Build history of the part. All positions in model axes, mm. A direction names the side the tool comes from. Coordinates: 2 decimals unless noted, no trailing zeros. Write each loop counter-clockwise with the first axis right and the second up, starting at its lowest first coordinate (ties: lowest second). Pieces come first, ordered by that corner, then holes. Notation, with made-up numbers: (16, 25) -> (57, 25) arc R25 cw to (57, 48) -> close; hole circle Ø1 at (73, 50.25). An arc over 180 degrees is marked (long way). Write each question's results on one line, items separated by ' | '. Start each with the question number.
Q1. Drop flat-ended pins along their axis: pin 1 Ø1.2 at (x, z) = (-10, 4) entering from -Y; pin 2 Ø4.5 at (x, y) = (-10.5, 7) entering from +Z; pin 3 Ø2 at (x, z) = (-3.5, 0.5) entering from +Y. Give the stop position or say it passes through.
Q2. Saw through at C-C on y = 1.5. Give the cut face in (x, z), and give its area (3 significant figures).
Q3. Drill centre lines: line 1 (Z direction, x = -1.25, y = 3.5); line 2 (Z direction, x = -14, y = 35); line 3 (Y direction, x = -9, z = -4). Where is each one in solid material? Low to high.
Q4. Tool access for faces 4 (the face through (-7.395, -9.491, 2.915)), 5 (the face through (-7, 4, 4.906)), 6 (the face through (0, -16, -3.3)): list every direction of +Z, -Z, +X, -X, +Y, -Y with a clear straight run to the whole face (end or side of a thin tool).
Q5. Two-plate mould, pull along Y, no slides. Class faces 1 (the face through (-7, 4, 3.406)), 2 (the face through (-7, 28, 2.406)), 3 (the face through (-7, -56.781, -5)): released by +Y, released by -Y, zero draft, split by the parting line, or undercut.
Q6. Saw through at D-D on z = -0.75. Give the cut face in (x, y).
Q7. Saw through at B-B on y = 20. Give the cut face in (x, z), and give its area (3 significant figures).
from build123d import *

# Parameters (mm, degrees)
F1_DEPTH = 15
F2_R     = 5
F3_W     = 19
F3_H     = 3.5
F4_DEPTH = 25
F5_R     = 5
F6_R     = 0.99999


# Not quite as in the source:
# - a fillet or chamfer is up to 0.001 mm smaller than in the source, because OpenCascade refuses the exact size


with BuildPart() as f1:
    # F0 (on Right) → F1 (new body)
    with BuildSketch(Plane.YZ):
        with BuildLine():
            Line((15.2185663986, 4.9061592609), (-8.3786299068, 4.9061592609))
            ThreePointArc((-8.3786299068, 4.9061592609), (-10.2743175345, 4.4284267718), (-11.7171893777, 3.10934347))
            Line((-11.7171893777, 3.10934347), (-15.1529792105, -2.0970249483))
            ThreePointArc((-15.1529792105, -2.0970249483), (-16.5958510537, -3.41610825), (-18.4915386814, -3.8938407391))
            Line((-18.4915386814, -3.8938407391), (-56.7814336014, -3.8938407391))
            Line((-56.7814336014, -3.8938407391), (-56.7814336014, -5.3938407391))
            Line((-56.7814336014, -5.3938407391), (-17.6842372959, -5.3938407391))
            ThreePointArc((-17.6842372959, -5.3938407391), (-15.7885496683, -4.91610825), (-14.3456778251, -3.5970249483))
            Line((-14.3456778251, -3.5970249483), (-10.9098879922, 1.60934347))
            ThreePointArc((-10.9098879922, 1.60934347), (-9.467016149, 2.9284267718), (-7.5713285214, 3.4061592609))
            Line((-7.5713285214, 3.4061592609), (15.2185663986, 3.4061592609))
            Line((15.2185663986, 3.4061592609), (15.2185663986, 4.9061592609))
        make_face()
    extrude(amount=-F1_DEPTH)

    # F2
    f2_edges = [f1.edges().sort_by_distance(p)[0] for p in [
        (-15, -56.781434, -4.643841),
        (0, -56.781434, -4.643841),
    ]]
    fillet(f2_edges, radius=F2_R)

    # F3 (on face) → F4 (join)
    with BuildSketch(Plane(origin=(0, 15.2185663986, 0), x_dir=(-1, 0, 0), z_dir=(0, 1, 0))):
        with Locations((7.5, 4.1561592609)):
            Rectangle(F3_W, F3_H)
    extrude(amount=F4_DEPTH)

    # F5
    f5_edges = [f1.edges().sort_by_distance(p)[0] for p in [
        (2, 40.218566, 4.156159),
        (-17, 40.218566, 4.156159),
    ]]
    fillet(f5_edges, radius=F5_R)

    # F6 (radius 1 in the source; OpenCascade refuses exactly that, so slightly less here)
    f6_edges = [f1.edges().sort_by_distance(p)[0] for p in [
        (-17, 25.218566, 5.906159),
        (-15.535534, 38.7541, 5.906159),
        (-7.5, 15.218566, 5.906159),
        (-7.5, 40.218566, 5.906159),
        (2, 25.218566, 5.906159),
        (0.535534, 38.7541, 5.906159),
        (2, 25.218566, 2.406159),
        (0.535534, 38.7541, 2.406159),
        (-7.5, 15.218566, 2.406159),
        (-7.5, 40.218566, 2.406159),
        (-17, 25.218566, 2.406159),
        (-15.535534, 38.7541, 2.406159),
        (2, 15.218566, 4.156159),
        (-17, 15.218566, 4.156159),
    ]]
    fillet(f6_edges, radius=F6_R)


solid = f1.part
Returned:
1) pin 1: stops at y = -11.51 | pin 2: stops at z = 4.91 | pin 3: stops at y = -10.98
2) outline: (-15, 3.41) -> (0, 3.41) -> (0, 4.91) -> (-15, 4.91) -> close | area: 22.5 mm2
3) line 1: z = 3.41 to 4.91 | line 2: z = 2.41 to 5.91 | line 3: y = -56.78 to -14.65
4) face 4: -Z, +X, -X | face 5: +Z, +X, -X, -Y | face 6: +Z, -Z, +X, -Y
5) face 1: undercut | face 2: zero draft | face 3: released by -Y
6) outline: (-15, -14.26) -> (0, -14.26) -> (0, -12.47) -> (-15, -12.47) -> close
7) outline: (-17, 3.41) arc R1 ccw to (-16, 2.41) -> (1, 2.41) arc R1 ccw to (2, 3.41) -> (2, 4.91) arc R1 ccw to (1, 5.91) -> (-16, 5.91) arc R1 ccw to (-17, 4.91) -> close | area: 65.6 mm2
